Source: three-view drawing plus pictorial views. Frame: mm from the lowest corner of the part. A direction names the side the tool comes from. Give positions to 0.01 mm unless a question says otherwise; leave off trailing zeros. Order: outer loops, then holes, each group sorted by start corner. A loop starts at its lowest first (then second) coordinate and runs counter-clockwise, first axis right, second up. Notation, with made-up numbers: M 22,58 L 64,58 A27 cw 64,91 Z; hole C -3.75,85 d7. An arc over 180 degrees is marked long. Use CSV: the item, a comma, the result in double quotes.
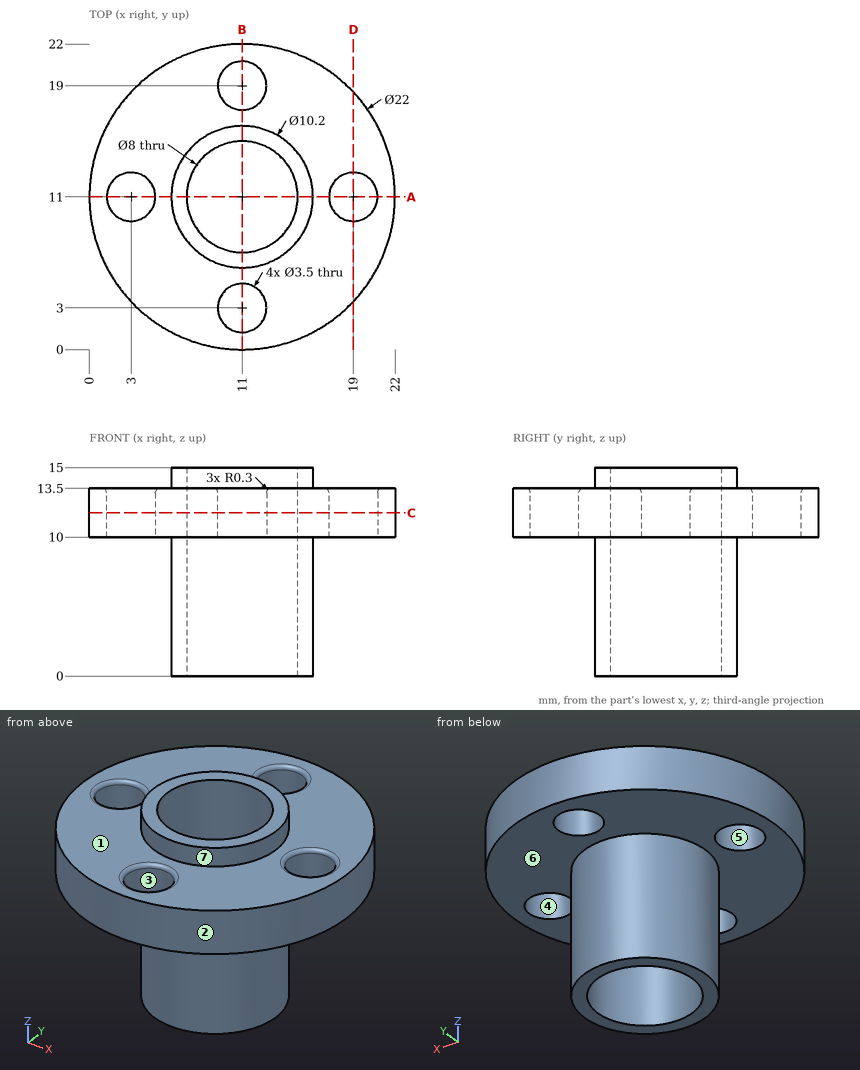
1. Pull-direction query (Y, two-part tool) for the marked faces 1, 2, 3 and 4; classes: +Y half, -Y half, draft (parallel to the pull), parting line (faces both ways), or undercut.
Answer:
face 1,"draft"
face 2,"parting line"
face 3,"undercut"
face 4,"undercut"
2. Section A-A, the plane y = 11. Return the cut outline in (x, z).
Answer:
outline,"M 0,10 L 1.25,10 L 1.25,13.2 A0.3 ccw 0.95,13.5 L 0,13.5 Z; M 4.75,10 L 5.9,10 L 5.9,0 L 7,0 L 7,15 L 5.9,15 L 5.9,13.5 L 5.05,13.5 A0.3 ccw 4.75,13.2 Z; M 15,0 L 16.1,0 L 16.1,10 L 17.25,10 L 17.25,13.2 A0.3 ccw 16.95,13.5 L 16.1,13.5 L 16.1,15 L 15,15 Z; M 20.75,10 L 22,10 L 22,13.5 L 21.05,13.5 A0.3 ccw 20.75,13.2 Z"
3. Section C-C, the plane z = 11.75. Return the cut outline in (x, y), plus the area to 3 significant figures.
Answer:
outline,"C 11,11 d22; hole C 3,11 d3.5; hole C 11,11 d8; hole C 11,3 d3.5; hole C 11,19 d3.5; hole C 19,11 d3.5"
area,"291 mm2"
4. Pin query (flat end, axial travel): pin 1 Ø8 at (y, z) = (6.5, 12.5) entering from -X; pin 2 Ø5 at (x, y) = (19.5, 17) entering from -Z; pin 3 Ø8 at (x, z) = (7, 11) entering from +Y; pin 4 Ø3 at (x, z) = (6.5, 13) entering from -Y. Return the tip coordinate at first contact, or that it passes through.
Answer:
pin 1,"x = 0.01"
pin 2,"z = 10"
pin 3,"y = 22"
pin 4,"y = 0.42"
5. Section D-D, the plane x = 19. Return the cut outline in (y, z).
Answer:
outline,"M 3.45,10 L 9.25,10 L 9.25,13.2 A0.3 ccw 8.95,13.5 L 3.45,13.5 Z; M 12.75,10 L 18.55,10 L 18.55,13.5 L 13.05,13.5 A0.3 ccw 12.75,13.2 Z"
6. Reachability of the marked faces 5, 6 and 7 from +Z, -Z, +X, -X, +Y, -Y: full face, straight path, thin tool, end or side. Return the list, or none.
Answer:
face 5,"+Z, -Z"
face 6,"-Z"
face 7,"+Z"
7. Line query: line 1 (Z direction, x = 2.75, y = 4.25); line 2 (X direction, y = 10.25, z = 12); line 3 (X direction, y = 9.75, z = 7). Output: solid intervals per line, ascending.
Answer:
line 1,"10 to 13.5"
line 2,"0.03 to 1.42, 4.58 to 7.07, 14.93 to 17.42, 20.58 to 21.97"
line 3,"6.06 to 7.2, 14.8 to 15.94"
